Geometry: final body of the model. Coordinates: model frame, mm. A direction names the side the tool comes from. Round coordinates to 2 decimals unless told otherwise and drop trailing zeros. Order: outer loops, then holes, each group sorted by start corner. A loop starts at its lowest first (then second) coordinate and runs counter-clockwise, first axis right, second up. Notation, with made-up numbers: M 32,0 L 80,0 A18 cw 80,19 Z; hole C 87,55.5 d3. An arc over 180 degrees is marked long. Put each result on its own line as item: value. Start each with the question number.
1) Material intervals for probe 1 along Y at (x, z) = (1.5, -4.5); probe 2 along X at (y, z) = (5.5, -5); probe 3 along Z at (x, y) = (13, 0.75), sorted ascending. Write a range as [from, to].
2) Access query for faces 1 (the flat face through (19.03, 3.958, -1.405)), 2 (the cylindrical face through (14.238, 3.958, 0.182)), 3 (the cylindrical face through (18.17, 7.7, -2.89)). Directions: +Z, -Z, +X, -X, +Y, -Y. A direction counts if a zero-diameter tool reaches every point of the face in a straight line with its end or side. Return the directions, or none.
3) Section B-B, the plane x = 12. Return loops of the section in (y, z), then the cut area to 3 significant figures.
4) First-contact query: P1, Ø2, axis at y = 6.5, z = -3.5, coming from the -X side; P2, Ø3, axis at y = 6.5, z = 0, coming from the +X side. Flat tips, straight axial feed; report the tip coordinate or a pass-through.
5) Section A-A, the plane y = 2. Return loops of the section in (x, z).
6) Section C-C, the plane z = 1. Return loops of the section in (x, y), then the cut area to 3 significant figures.
from build123d import *

# Parameters (mm, degrees)
BOSS_EXTRUDE1_DEPTH = 1
BOSS_EXTRUDE2_DEPTH = 7
LPATTERN1_COUNT     = 2
LPATTERN1_PITCH     = 14
FILLET3_R           = 1
SKETCH3_R           = 1
CUT_EXTRUDE1_DEPTH  = 29.970188425


with BuildPart() as part:
    # Sketch1 → Boss-Extrude1 (new body)
    with BuildSketch(Plane(origin=(0, 0, 0), x_dir=(1, 0, 0), z_dir=(0, 1, 0))):
        with BuildLine():
            Line((0, -3.701311317), (15.650619727, -3.701311317))
            ThreePointArc((15.650619727, -3.701311317), (16.168257817, -3.633162969), (16.650619727, -3.433362124))
            Line((16.650619727, -3.433362124), (25.008301572, 1.391947739))
            ThreePointArc((25.008301572, 1.391947739), (26.732838106, 5.555347227), (23.157645914, 8.298688683))
            Line((23.157645914, 8.298688683), (7.507026187, 8.298688683))
            ThreePointArc((7.507026187, 8.298688683), (6.989388097, 8.230540336), (6.507026187, 8.030739491))
            Line((6.507026187, 8.030739491), (-1.850655658, 3.205429628))
            ThreePointArc((-1.850655658, 3.205429628), (-3.575192192, -0.957969861), (0, -3.701311317))
        make_face()
    extrude(amount=BOSS_EXTRUDE1_DEPTH)

    # Sketch2 → Boss-Extrude2 (add)
    with BuildSketch(Plane(origin=(0, 1, 0), x_dir=(1, 0, 0), z_dir=(0, 1, 0))):
        with BuildLine():
            Line((15.614721342, -0.567336721), (22.542924572, 3.432663279))
            ThreePointArc((22.542924572, 3.432663279), (22.908949976, 4.798688683), (21.542924572, 5.164714087))
            Line((21.542924572, 5.164714087), (14.614721342, 1.164714087))
            ThreePointArc((14.614721342, 1.164714087), (14.248695938, -0.201311317), (15.614721342, -0.567336721))
        make_face()
    boss_extrude2 = extrude(amount=BOSS_EXTRUDE2_DEPTH)

    # LPattern1: Boss-Extrude2 ×2
    with Locations(*[(-i * LPATTERN1_PITCH, 0, 0) for i in range(1, LPATTERN1_COUNT)]):
        add(boss_extrude2)

    # Fillet3
    fillet3_edges = [part.edges().sort_by_distance(p)[0] for p in [
        (18.078822957, 8, -3.164714087),
        (19.078822957, 8, -1.432663279),
        (22.908949976, 8, -4.798688683),
        (14.248695938, 8, 0.201311317),
        (4.078822957, 8, -3.164714087),
        (5.078822957, 8, -1.432663279),
        (8.908949976, 8, -4.798688683),
        (0.248695938, 8, 0.201311317),
    ]]
    fillet(fillet3_edges, radius=FILLET3_R - 0.0001)  # a hair under: the kernel refuses the full size

    # Sketch3 → Cut-Extrude1 (cut, through all)
    with BuildSketch(Plane(origin=(0, 1, 0), x_dir=(1, 0, 0), z_dir=(0, 1, 0))):
        with Locations(Location((13.489388097, 6.298688683, 0), (0, 0, 270))):
            Circle(SKETCH3_R)
    extrude(amount=-CUT_EXTRUDE1_DEPTH, mode=Mode.SUBTRACT)


solid = part.part
Result sheet:
1. probe 1: y = [0, 1]
1. probe 2: x = [7.26, 8.76], [21.26, 22.76]
1. probe 3: z = [-8.3, -7.17], [-5.43, 3.7]
2. face 1: +Z, +X, +Y
2. face 2: +Y
2. face 3: -Z, +Y
3. outline: M 0,-8.3 L 1,-8.3 L 1,3.7 L 0,3.7 Z
3. area: 12.0 mm2
4. P1: stops at x = 2.93
4. P2: stops at x = 19.2
5. outline: M 0.61,-1.16 L 7.54,-5.16 A1 ccw 8.54,-3.43 L 1.61,0.57 A1 ccw Z; M 14.61,-1.16 L 21.54,-5.16 A1 ccw 22.54,-3.43 L 15.61,0.57 A1 ccw Z
6. outline: M -3.56,0 L 20.87,0 L 20.87,1 L -3.56,1 Z
6. area: 24.4 mm2
